Autodesk Inventor part; units mm, degrees
ref_plane "YZ Plane" through (0, 0, 0) normal (1, 0, 0) x (0, 1, 0)
ref_plane "XZ Plane" through (0, 0, 0) normal (0, 1, 0) x (-1, 0, 0)
ref_plane "XY Plane" through (0, 0, 0) normal (0, 0, 1) x (1, 0, 0)
sketch "Sketch1" plane through (0, 0, 0) normal (0, 0, 1) x (1, 0, 0)
  circle A0 centre (-4.8443, 5.8204) radius 6.35 construction
  arc A1 (-6.7493, 12.1704) -> (-2.9393, 12.1704) centre (-4.8443, 12.3033) ccw
  line L0 (-8.5105, 12.1704) -> (-6.7493, 12.1704)
  line L1 (-2.9393, 12.1704) -> (-1.1781, 12.1704)
  arc A2 (-0.2975, 10.6452) -> (1.6075, 7.3457) centre (0.7701, 9.0619) ccw
  arc A3 (1.6075, 4.2952) -> (-0.2975, 0.9957) centre (0.7701, 2.579) ccw
  arc A4 (-2.9393, -0.5296) -> (-6.7493, -0.5296) centre (-4.8443, -0.6625) ccw
  arc A5 (-9.3911, 0.9957) -> (-11.2961, 4.2952) centre (-10.4586, 2.579) ccw
  arc A6 (-11.2961, 7.3457) -> (-9.3911, 10.6452) centre (-10.4586, 9.0619) ccw
  line L2 (-12.1766, 5.8204) -> (-11.2961, 7.3457)
  line L3 (-8.5105, -0.5296) -> (-9.3911, 0.9957)
  line L4 (-1.1781, -0.5296) -> (-2.9393, -0.5296)
  line L5 (2.4881, 5.8204) -> (1.6075, 4.2952)
  line L6 (-1.1781, 12.1704) -> (-0.2975, 10.6452)
  line L7 (-9.3911, 10.6452) -> (-8.5105, 12.1704)
  line L8 (-11.2961, 4.2952) -> (-12.1766, 5.8204)
  line L9 (-6.7493, -0.5296) -> (-8.5105, -0.5296)
  line L10 (-0.2975, 0.9957) -> (-1.1781, -0.5296)
  line L11 (1.6075, 7.3457) -> (2.4881, 5.8204)
  point P0 (0, 0)
  point P1 (-4.8443, -0.5296)
  point P2 (-4.8443, 12.1704)
  point P3 (0.655, 8.9954)
  point P4 (0.655, 2.6454)
  point P5 (-4.8443, -0.5296)
  point P6 (-10.3436, 2.6454)
  point P7 (-10.3436, 8.9954)
  point P8 (-0.2975, 10.6452)
  point P9 (-9.3911, 10.6452)
  point P10 (-11.2961, 4.2952)
  point P11 (-9.3911, 0.9957)
  point P12 (-6.7493, -0.5296)
  point P13 (-2.9393, -0.5296)
  point P14 (1.6075, 7.3457)
  dimension "d2" = 12.7
  dimension "d7" = 360
  dimension "d11" = 360
  dimension "d15" = 360
extrude "Extrusion1" add sketch "Sketch1" along normal blind 558.8
sketch "Sketch2" plane through (0, 0, 558.8) normal (0, 0, 1) x (1, 0, 0)
  circle A0 centre (-4.8443, 5.8204) radius 2.9337
  line L0 (-8.5105, -0.5296) -> (-6.7493, -0.5296)
  line L1 (-8.5105, 12.1704) -> (-8.5105, -0.5296) construction
  line L2 (-1.1781, 12.1704) -> (-2.9393, 12.1704)
  line L3 (-2.9393, -0.5296) -> (-1.1781, -0.5296)
  line L4 (-1.1781, 12.1704) -> (-1.1781, -0.5296) construction
  line L5 (-4.8443, 9.4005) -> (-4.8443, 3.0295) construction
  point P0 (0, 0)
  dimension "d19" = 6.35
  dimension "d20" = 5.8674
extrude "Extrusion2" cut sketch "Sketch2" against normal blind 558.8
equation "\"d17\" = d23"
equation "\"d21\" = d23"
equation "\"d23\" = 558.8"
properties part number "Churro 22in"
Can you work these out from the model? Positions are in its coordinate system, mm. Coordinates: 2 decimals unless noted, no trailing zeros. Loops run counter-clockwise (first coordinate to the right, second up) from the corner with the lowest first, then second, coordinate; pieces in that order, holes last.
1) I need wall thicknesses on probe 1 along Y at (x, z) = (-4.75, 402); probe 2 along Y at (x, z) = (-4.5, 48.5); probe 3 along Y at (x, z) = (-8.75, 527). Which ranges of each line are inside material? Lowest first, please.
2) For pin 1 (3 mm diameter, centred on y = 7.5, z = 360, fed in from -X); pin 2 (1 mm diameter, centred on x = -9.5, y = 2.5, fed in from +Z); pin 3 (3 mm diameter, centred on y = 9.5, z = 176, fed in from +X), each with a flat end and sliding along its axis, tell me the tip position at first contact or that it passes through.
3) Imagine slicing it at A-A on z = 419.5. List the corners of the cut face in (x, y) for me.
Completed:
1. probe 1: y = 1.24 to 2.89, 8.75 to 10.4
1. probe 2: y = 1.22 to 2.91, 8.73 to 10.42
1. probe 3: y = -0.11 to 1.73, 3.43 to 8.21, 9.91 to 11.76
2. pin 1: stops at x = -12.07
2. pin 2: passes through
2. pin 3: stops at x = -0.3
3. outline: (-12.18, 5.82) - (-11.3, 4.3) arc R1.91 cw to (-9.39, 1) - (-8.51, -0.53) - (-6.75, -0.53) arc R1.91 cw to (-2.94, -0.53) - (-1.18, -0.53) - (-0.3, 1) arc R1.91 cw to (1.61, 4.3) - (2.49, 5.82) - (1.61, 7.35) arc R1.91 cw to (-0.3, 10.65) - (-1.18, 12.17) - (-2.94, 12.17) arc R1.91 cw to (-6.75, 12.17) - (-8.51, 12.17) - (-9.39, 10.65) arc R1.91 cw to (-11.3, 7.35) - close; hole circle Ø5.87 at (-4.84, 5.82)
